Source: CAD feature listing. Evaluate the final solid. Frame: model axes, mm. A direction names the side the tool comes from. Give positions to 0.01 mm unless a question says otherwise; leave off trailing zeros. Write each loop counter-clockwise with the first axis right and the second up, starting at its lowest first coordinate (ties: lowest second). Pieces come first, ordered by that corner, then holes. Notation, with made-up numbers: M 54,77.25 L 80,77.25 A22 cw 80,116.25 Z; hole C 54,-0.5 d7. An arc over 180 degrees is marked long. Answer as a JSON object with one key per item and string values. Group by question number.
```python
from build123d import *

# Parameters (mm, degrees)
F0_W     = 40
F0_H     = 40
F0_W_2   = 35
F0_H_2   = 35
F1_DEPTH = 6
F2_DEPTH = 2
F3_W     = 2.5
F3_H     = 30
F4_DEPTH = 2


with BuildPart() as f1:
    # F0 (on Front) → F1 (new body)
    with BuildSketch(Plane.XZ):
        Rectangle(F0_W, F0_H)
        Rectangle(F0_W_2, F0_H_2, mode=Mode.SUBTRACT)
    extrude(amount=F1_DEPTH)

    # F0 (on Front) → F2 (join)
    with BuildSketch(Plane.XZ):
        Rectangle(F0_W_2, F0_H_2)
    extrude(amount=F2_DEPTH)

    # F3 (on face) → F4 (join)
    with BuildSketch(Plane.XZ.offset(6)):
        Polygon((-17.5, 17.5), (-17.5, 15), (-15, 15), (15, 15), (17.5, 15), (17.5, 17.5), align=None)
        with Locations((-16.25, 0)):
            Rectangle(F3_W, F3_H)
        Polygon((-15, -15), (-17.5, -15), (-17.5, -17.5), (15, -17.5), (15, -15), align=None)
        Polygon((17.5, 15), (15, 15), (15, -15), (15, -17.5), (17.5, -17.5), align=None)
    extrude(amount=-F4_DEPTH)


solid = f1.part
```
(1) Section B-B, the plane x = -16.5. Return loops of the section in (y, z).
(2) Ray query, L1, parallel to X at y = -4.75, z = -13.5; L2, parallel to X at y = -3.35, z = -5.5; L3, parallel to Y at x = 7.5, z = 16. Return the intervals inside material, ascending. Write a range as [from, to].
(3) Pull-direction query (Z, two-part tool) for faces 1 (the flat face through (0, -2, 0)), 2 (the flat face through (0, -3, -20)), 3 (the flat face through (-20, -3, 0)); classes: pulls with the +Z half, pulls with the -Z half, needs draft (parallel to the pull), parting line crosses it, or undercut.
(4) Access query for faces 4 (the flat face through (-18, -6, 0)), 5 (the flat face through (15, -5, 0)), 6 (the flat face through (17.5, -3, 0)). Directions: +Z, -Z, +X, -X, +Y, -Y. A direction counts if a zero-diameter tool reaches every point of the face in a straight line with its end or side. Return the directions, or none.
(5) Section D-D, the plane x = -5. Return loops of the section in (y, z), plus the area to 3 significant figures.
(6) Section C-C, the plane z = 12.5. Return loops of the section in (x, y).
(7) Section A-A, the plane y = -4.65. Return loops of the section in (x, z), plus the area to 3 significant figures.
Reported:
{
 "1": {"outline": "M -6,-20 L 0,-20 L 0,20 L -6,20 Z; hole M -4,-17.5 L -2,-17.5 L -2,17.5 L -4,17.5 Z"},
 "2": {"L1": "x = [-20, -15], [15, 20]", "L2": "x = [-20, -17.5], [17.5, 20]", "L3": "y = [-6, -4], [-2, 0]"},
 "3": {"face 1": "undercut", "face 2": "pulls with the -Z half", "face 3": "needs draft"},
 "4": {"face 4": "+Z, -Z, +X, -X, -Y", "face 5": "-Y", "face 6": "none"},
 "5": {"outline": "M -6,-20 L 0,-20 L 0,20 L -6,20 L -6,15 L -4,15 L -4,17.5 L -2,17.5 L -2,-17.5 L -4,-17.5 L -4,-15 L -6,-15 Z", "area": "110 mm2"},
 "6": {"outline": "M -20,-6 L -15,-6 L -15,-4 L -17.5,-4 L -17.5,-2 L 17.5,-2 L 17.5,-4 L 15,-4 L 15,-6 L 20,-6 L 20,0 L -20,0 Z"},
 "7": {"outline": "M -20,-20 L 20,-20 L 20,20 L -20,20 Z; hole M -15,-15 L 15,-15 L 15,15 L -15,15 Z", "area": "700 mm2"}
}
